Could you check a few things on this drawing? It's one solid part, dimensions in mm from its lowest x, y, z. A direction names the side the tool comes from. Give positions to 0.01 mm unless a question says otherwise; leave off trailing zeros. Order: outer loops, then holes, each group sorted by start corner. A loop starts at its lowest first (then second) coordinate and runs counter-clockwise, first axis right, second up. Notation, with made-up numbers: M 68.25,56 L 91.25,56 A28 cw 91.25,76 Z; hole C 76,19.5 d10. An arc over 180 degrees is marked long. Use one line per item in the form item = value. Start each with the question number.
1. I want a section at A-A, the plane y = 22. List the corners of the cut face in (x, z) for me.
2. I want a section at C-C, the plane z = 4. List the corners of the cut face in (x, y) for me.
3. I want a section at D-D, the plane x = 93.5. List the corners of the cut face in (y, z) for me.
4. I want a section at B-B, the plane y = 47. List the corners of the cut face in (x, z) for me.
5. For the marked faces 1, 2 and 3, which set-ups out of +Z, -Z, +X, -X, +Y, -Y let a thin tool reach every point of the face, with its end or its side?
6. Will these pins go through, and if not, where does the flat tip stop? P1, Ø4, axis at y = 16.5, z = 54.5, coming from the -X side; P2, Ø4, axis at x = 5, z = 57.5, coming from the -Y side; P3, Ø8, axis at x = 85, z = 42.5, coming from the -Y side.
7. I need wall thicknesses on L1, parallel to Y at x = 33, z = 13; L2, parallel to X at y = 30, z = 11.5. Which ranges of each line are inside material? Lowest first, please.
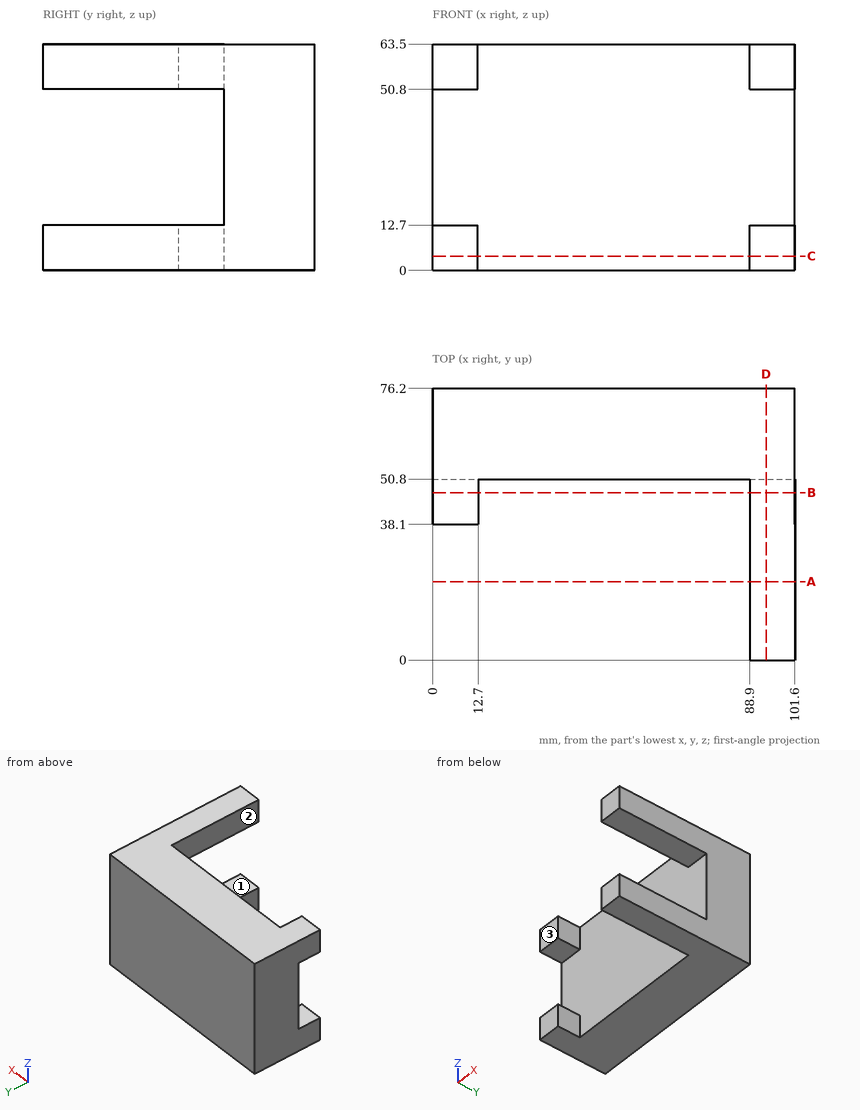
Check result:
q1.outline = M 88.9,0 L 101.6,0 L 101.6,12.7 L 88.9,12.7 Z; M 88.9,50.8 L 101.6,50.8 L 101.6,63.5 L 88.9,63.5 Z
q2.outline = M 0,38.1 L 12.7,38.1 L 12.7,50.8 L 88.9,50.8 L 88.9,0 L 101.6,0 L 101.6,76.2 L 0,76.2 Z
q3.outline = M 0,0 L 76.2,0 L 76.2,63.5 L 0,63.5 L 0,50.8 L 50.8,50.8 L 50.8,12.7 L 0,12.7 Z
q4.outline = M 0,0 L 12.7,0 L 12.7,12.7 L 0,12.7 Z; M 0,50.8 L 12.7,50.8 L 12.7,63.5 L 0,63.5 Z; M 88.9,0 L 101.6,0 L 101.6,12.7 L 88.9,12.7 Z; M 88.9,50.8 L 101.6,50.8 L 101.6,63.5 L 88.9,63.5 Z
q5.face_1 = +X, -X, -Y
q5.face_2 = +Z, -Z, -Y
q5.face_3 = +Z, -Z, -X, -Y
q6.P1 = 88.9
q6.P2 = 38.1
q6.P3 = 50.8
q7.L1 = 50.8 to 76.2
q7.L2 = 88.9 to 101.6
